from build123d import *

# Parameters (mm, degrees)
SKETCH1_W           = 101.6
SKETCH1_H           = 50.8
BOSS_EXTRUDE1_DEPTH = 50.8
BOSS_EXTRUDE2_DEPTH = 101.6
CUT_EXTRUDE1_DEPTH  = 101.6
SHELL1_T            = -2.54
SKETCH4_W           = 101.6
SKETCH4_H           = 2.54
BOSS_EXTRUDE3_DEPTH = 12.7
CUT_EXTRUDE2_DEPTH  = 2.54
LPATTERN1_COUNT     = 11
LPATTERN1_PITCH     = 9.652


with BuildPart() as part:
    # Sketch1 → Boss-Extrude1 (new body)
    with BuildSketch(Plane.XY):
        with Locations((50.8, 25.4)):
            Rectangle(SKETCH1_W, SKETCH1_H)
    extrude(amount=-BOSS_EXTRUDE1_DEPTH)

    # Sketch2 → Boss-Extrude2 (add)
    with BuildSketch(Plane.ZY):
        with BuildLine():
            Line((-50.8, 50.8), (-50.8, 0))
            ThreePointArc((-50.8, 0), (-76.2, 25.4), (-50.8, 50.8))
        make_face()
    extrude(amount=-BOSS_EXTRUDE2_DEPTH)

    # Sketch3 → Cut-Extrude1 (cut)
    with BuildSketch(Plane.ZY):
        Polygon((0, 0), (-25.4, 50.8), (0, 50.8), align=None)
    extrude(amount=-CUT_EXTRUDE1_DEPTH, mode=Mode.SUBTRACT)

    # Shell1
    shell1_openings = [part.faces().sort_by_distance(p)[0] for p in [
        (50.8, 25.4, -12.7),
    ]]
    offset(amount=SHELL1_T, openings=shell1_openings, kind=Kind.INTERSECTION)

    # Sketch4 → Boss-Extrude3 (add)
    with BuildSketch(Plane.XY.offset(-2.54)):
        with Locations((50.8, 1.27)):
            Rectangle(SKETCH4_W, SKETCH4_H)
    extrude(amount=BOSS_EXTRUDE3_DEPTH)

    # Sketch5 → Cut-Extrude2 (cut)
    with BuildSketch(Plane(origin=(0, 2.54, 0), x_dir=(1, 0, 0), z_dir=(0, 1, 0))):
        Polygon((0, 0), (4.208409794, -10.16), (0, -10.16), align=None)
        Polygon((5.478409794, -10.16), (9.686819587, 0), (9.686819587, -10.16), align=None)
    cut_extrude2 = extrude(amount=-CUT_EXTRUDE2_DEPTH, mode=Mode.SUBTRACT)

    # LPattern1: Cut-Extrude2 ×11
    with Locations(*[(i * LPATTERN1_PITCH, 0, 0) for i in range(1, LPATTERN1_COUNT)]):
        add(cut_extrude2, mode=Mode.SUBTRACT)


solid = part.part
Geometry: final body of the model. Coordinates: model frame, mm. A direction names the side the tool comes from. Round coordinates to 2 decimals unless told otherwise and drop trailing zeros. Order: outer loops, then holes, each group sorted by start corner. A loop starts at its lowest first (then second) coordinate and runs counter-clockwise, first axis right, second up. Notation, with made-up numbers: (72, 71.25) -> (82, 71.25) arc R37 ccw to (82, 110.25) -> close; hole circle Ø9 at (42.25, -26). An arc over 180 degrees is marked (long way). Put each result on its own line as item: value. Start each with the question number.
Q1. Section B-B on y = 25.4. Return the cut outline in (x, z).
Q2. Section C-C on x = 12. Return the cut outline in (y, z), and give its area (3 significant figures).
Q3. Section A-A on z = -44. Return the cut outline in (x, y), and give its area (3 significant figures).
Q4. Section D-D on z = -66.5. Return the cut outline in (x, y), and give its area (3 significant figures).
Q5. Pull-direction query (X, two-part tool) for faces 4 (the flat face through (36.492, 1.288, 5.193)), 5 (the flat face through (26.84, 1.29, 5.19)), 6 (the flat face through (2.075, 1.288, 5.009)), 7 (the flat face through (50, 0, -21)); classes: +X half, -X half, draft (parallel to the pull), parting line (faces both ways), or undercut.
Q6. Line query: probe 1 along X at (y, z) = (11.5, -26); probe 2 along Y at (x, z) = (21, -27); probe 3 along Y at (x, z) = (85.5, -7). Output: solid intervals per line, ascending.
Q7. First-contact query: pin 1 (2 mm diameter, centred on x = 25, y = 31.5, fed in from +Z); pin 2 (4 mm diameter, centred on x = 20, y = 25, fed in from +Z); pin 3 (1.5 mm diameter, centred on x = 45.5, y = 20.5, fed in from +Z). Flat tips, straight axial feed; report the tip coordinate or a pass-through.
Q8. Reachability of faces 1 (the flat face through (31.048, 1.288, 5.051)), 2 (the flat face through (0, 25, -39)), 3 (the flat face through (50, 48.26, -37)) from +Z, -Z, +X, -X, +Y, -Y: full face, straight path, thin tool, end or side. Return the list, or none.
Ans:
1. outline: (0, -76.2) -> (101.6, -76.2) -> (101.6, -12.7) -> (99.06, -12.7) -> (99.06, -73.66) -> (2.54, -73.66) -> (2.54, -12.7) -> (0, -12.7) -> close
2. outline: (0, -50.8) arc R25.4 ccw to (50.8, -50.8) -> (50.8, -25.4) -> (48.26, -24.13) -> (48.26, -50.8) arc R22.86 cw to (2.54, -50.8) -> (2.54, 5.67) -> (0, 5.67) -> close
2. area: 402 mm2
3. outline: (0, 0) -> (101.6, 0) -> (101.6, 50.8) -> (0, 50.8) -> close; hole (2.54, 2.54) -> (99.06, 2.54) -> (99.06, 48.26) -> (2.54, 48.26) -> close
3. area: 748 mm2
4. outline: (0, 5.43) -> (101.6, 5.43) -> (101.6, 45.37) -> (0, 45.37) -> close; hole (2.54, 8.78) -> (99.06, 8.78) -> (99.06, 42.02) -> (2.54, 42.02) -> close
4. area: 850 mm2
5. face 4: undercut
5. face 5: undercut
5. face 6: -X half
5. face 7: draft
6. probe 1: x = 0 to 2.54, 99.06 to 101.6
6. probe 2: y = 0 to 2.54, 48.26 to 50.8
6. probe 3: y = 0 to 2.54
7. pin 1: stops at z = -72.53
7. pin 2: stops at z = -73.53
7. pin 3: stops at z = -72.95
8. face 1: +Z, +Y, -Y
8. face 2: +Z, -Z, -X, +Y, -Y
8. face 3: +Z
